Could you check a few things on this model? Use its own coordinates, in mm. Round coordinates to 2 decimals unless told otherwise and drop trailing zeros. Loops run counter-clockwise (first coordinate to the right, second up) from the corner with the lowest first, then second, coordinate; pieces in that order, holes last. Notation, with made-up numbers: (-29.5, 3.5) - (22.5, 3.5) arc R22 cw to (22.5, 37.5) - close; hole circle Ø2 at (45, 83). An arc over 180 degrees is marked (long way). Use one line per item in the form item = value.
```python
from build123d import *

# Parameters (mm, degrees)
SKETCH1_W                      = 60
SKETCH1_H                      = 30
SKETCH1_R                      = 2.3
BOSS_EXTRUDE1_DEPTH            = 4.6
CUT_EXTRUDE1_REACH             = 35.855
SKETCH2_R                      = 1.875
CUT_EXTRUDE1_DIRECTION_2_DEPTH = 34.854984862


with BuildPart() as part:
    # Sketch1 → Boss-Extrude1 (new body)
    with BuildSketch(Plane.XY):
        Rectangle(SKETCH1_W, SKETCH1_H)
        with Locations((-13.800714267, 9.000714267)):
            Circle(SKETCH1_R, mode=Mode.SUBTRACT)
        with Locations((5.999285733, 9.000714267)):
            Circle(SKETCH1_R, mode=Mode.SUBTRACT)
        with Locations((20, -5)):
            Circle(SKETCH1_R, mode=Mode.SUBTRACT)
    extrude(amount=BOSS_EXTRUDE1_DEPTH)

    # Sketch2 → Cut-Extrude1 (cut, up to next)
    with BuildSketch(Plane.XY.offset(4.6), mode=Mode.PRIVATE) as cut_extrude1_sk1:
        with Locations(Location((-27.5, -7.5, 0), (0, 0, 180))):
            Circle(SKETCH2_R)
    cut_extrude1_tool1 = extrude(cut_extrude1_sk1.sketch, amount=-CUT_EXTRUDE1_REACH, mode=Mode.PRIVATE) & part.part
    # Sketch2 → Cut-Extrude1 (cut, up to next)
    with BuildSketch(Plane.XY.offset(4.6), mode=Mode.PRIVATE) as cut_extrude1_sk2:
        with Locations(Location((27.5, 7.5, 0), (0, 0, 180))):
            Circle(SKETCH2_R)
    cut_extrude1_tool2 = extrude(cut_extrude1_sk2.sketch, amount=-CUT_EXTRUDE1_REACH, mode=Mode.PRIVATE) & part.part
    add(cut_extrude1_tool1.solids().sort_by_distance((-27.5, -7.5, 4.6))[0], mode=Mode.SUBTRACT)
    add(cut_extrude1_tool2.solids().sort_by_distance((27.5, 7.5, 4.6))[0], mode=Mode.SUBTRACT)

    # Sketch2 → Cut-Extrude1 direction 2 (cut)
    with BuildSketch(Plane.XY.offset(4.6)):
        with Locations(Location((-27.5, -7.5, 0), (0, 0, 180))):
            Circle(SKETCH2_R)
        with Locations(Location((27.5, 7.5, 0), (0, 0, 180))):
            Circle(SKETCH2_R)
    extrude(amount=CUT_EXTRUDE1_DIRECTION_2_DEPTH, mode=Mode.SUBTRACT)


solid = part.part
```
1. For P1, Ø4, axis at x = 20, y = -5, coming from the -Z side, with a flat end and sliding along its axis, tell me the tip position at first contact or that it passes through.
Solution:
P1 = through
2. If we section it at A-A, the plane x = 20: Write out the boundary of the cut face in (y, z), plus the area to 3 significant figures.
Solution:
outline = (-15, 0) - (-7.3, 0) - (-7.3, 4.6) - (-15, 4.6) - close; (-2.7, 0) - (15, 0) - (15, 4.6) - (-2.7, 4.6) - close
area = 117 mm^2
3. If we section it at C-C, the plane z = 1.3: Write out the boundary of the cut face in (x, y) (3 decimals).
Solution:
outline = (-30, -15) - (30, -15) - (30, 15) - (-30, 15) - close; hole circle Ø3.75 at (-27.5, -7.5); hole circle Ø4.6 at (-13.801, 9.001); hole circle Ø4.6 at (5.999, 9.001); hole circle Ø4.6 at (20, -5); hole circle Ø3.75 at (27.5, 7.5)
4. If we section it at B-B, the plane y = -5: Write out the boundary of the cut face in (x, z), plus the area to 3 significant figures.
Solution:
outline = (-30, 0) - (17.7, 0) - (17.7, 4.6) - (-30, 4.6) - close; (22.3, 0) - (30, 0) - (30, 4.6) - (22.3, 4.6) - close
area = 255 mm^2
5. Please list where these lines run through material, in increasing order: line 1 along Y through (x, z) = (20, 1.45); line 2 along Y through (x, z) = (-27.5, 3) (3 decimals); line 3 along X through (y, z) = (-7.5, 3.45) (3 decimals).
Solution:
line_1 = -15 to -7.3, -2.7 to 15
line_2 = -15 to -9.375, -5.625 to 15
line_3 = -30 to -29.375, -25.625 to 30
6. We'd pull the mould along X, two halves only. Please class faces 1 (the face through (22.194, -4.309, 2.268)), 2 (the face through (-30, 0, 2)), 3 (the face through (0, 0, 4.6)), 4 (the face through (25.71, 6.94, 2.33)): +X half, -X half, draft (parallel to the pull), parting line (faces both ways), or undercut.
Solution:
face_1 = undercut
face_2 = -X half
face_3 = draft
face_4 = undercut
